Check sheet for the modelled part. Datum: model origin and axes. Units: mm. A direction names the side the tool comes from. Round coordinates to 2 decimals unless told otherwise and drop trailing zeros. Write each loop counter-clockwise with the first axis right and the second up, starting at its lowest first coordinate (ties: lowest second). Pieces come first, ordered by that corner, then holes. Notation, with made-up numbers: M 5.25,54.5 L 30.25,54.5 A17 cw 30.25,82.5 Z; hole C 83.25,40.5 d9. An arc over 180 degrees is marked long. One line per item, written item: value.
from build123d import *

# Parameters (mm, degrees)
F0_W          = 28.3
F0_H          = 28.2685337434
F0_R          = 1.5
F1_DEPTH      = 5
F2_W          = 45
F2_H          = 10
F3_DEPTH      = 5
F4_W          = 10
F4_H          = 25
F5_DEPTH      = 35
F7_DEPTH      = 30
F7_DEPTH_BACK = 10
F8_T1_DEPTH   = 51.2903171605
F8_T3_DEPTH   = 50.8819045103
F8_T5_DEPTH   = 44.5915873497
F8_T7_DEPTH   = 15.5291427062
F8_T9_DEPTH   = 33.4838731358
F8_T11_DEPTH  = 29.4646352493
F8_T13_DEPTH  = 15
F8_T15_DEPTH  = 17.5
F8_T20_DEPTH  = 5
F8_T26_DEPTH  = 5
F8_S31_W      = 5
F8_S31_H      = 5
F8_T32_DEPTH  = 5
F8_S37_W      = 5
F8_S37_H      = 5
F8_T38_DEPTH  = 5


# Not quite as in the source:
# - a fillet or chamfer that OpenCascade refuses, or shapes differently, is made with other operations: its cross-section is extruded or revolved along the edge and cut away or added


with BuildPart() as f1:
    # F0 (on Top) → F1 (new body)
    with BuildSketch(Plane.XY):
        Rectangle(F0_W, F0_H)
        with Locations((-10.4845586502, -10.7272564019)):
            Circle(F0_R, mode=Mode.SUBTRACT)
        with Locations((10.7272564019, -10.4845586502)):
            Circle(F0_R, mode=Mode.SUBTRACT)
        with Locations((-10.7272564019, 10.4845586502)):
            Circle(F0_R, mode=Mode.SUBTRACT)
        with Locations((10.4845586502, 10.7272564019)):
            Circle(F0_R, mode=Mode.SUBTRACT)
    extrude(amount=F1_DEPTH)

    # F2 (on face) → F3 (join)
    with BuildSketch(Plane.XY.offset(5)):
        with Locations((8.35, 0)):
            Rectangle(F2_W, F2_H)
    extrude(amount=F3_DEPTH)

    # F4 (on face) → F5 (join)
    with BuildSketch(Plane(origin=(0, 0, 5), x_dir=(1, 0, 0), z_dir=(0, 0, -1))):
        with Locations((25.85, 0)):
            Rectangle(F4_W, F4_H)
    extrude(amount=-F5_DEPTH)

    # F6 (on face) → F7 (join, two sides)
    with BuildSketch(Plane(origin=(20.85, 0, 0), x_dir=(0, -1, 0), z_dir=(-1, 0, 0))) as f7_sk:
        Polygon((-12.5, 50), (-12.5, 40), (12.5, 40), (12.5, 43.3012701892), align=None)
    extrude(amount=F7_DEPTH)
    extrude(f7_sk.sketch, amount=-F7_DEPTH_BACK)

    # F8: fillet of radius 5 on 9 edges, made by hand

    # F8_s2 → F8_t1 (cut)
    with BuildSketch(Plane.YZ.offset(-25.4403171605)):
        with BuildLine():
            ThreePointArc((6.2059047745, 48.3135022672), (10.543807145, 47.4506398373), (12.5, 43.4838731358))
            Line((12.5, 43.4838731358), (12.5, 50))
            Line((12.5, 50), (6.2059047745, 48.3135022672))
        make_face()
    extrude(amount=F8_T1_DEPTH, mode=Mode.SUBTRACT)

    # F8_s4 → F8_t3 (cut)
    with BuildSketch(Plane(origin=(0, -12.911414055, -3.4596029692), x_dir=(1, 0, 0), z_dir=(0, 0.9659258263, 0.2588190451))):
        with BuildLine():
            ThreePointArc((-9.15, -40.0610532507), (-7.6855339059, -43.5965871566), (-4.15, -45.0610532507))
            Line((-4.15, -45.0610532507), (-9.15, -45.0610532507))
            Line((-9.15, -45.0610532507), (-9.15, -40.0610532507))
        make_face()
    extrude(amount=F8_T3_DEPTH, mode=Mode.SUBTRACT)

    # F8_s6 → F8_t5 (cut)
    with BuildSketch(Plane.YZ.offset(-18.7415873497)):
        with BuildLine():
            ThreePointArc((-12.5, 39.4646352493), (-11.4667667015, 42.5084423944), (-8.7940952255, 44.2942643808))
            Line((-8.7940952255, 44.2942643808), (-12.5, 43.3012701892))
            Line((-12.5, 43.3012701892), (-12.5, 39.4646352493))
        make_face()
    extrude(amount=F8_T5_DEPTH, mode=Mode.SUBTRACT)

    # F8_s8 → F8_t7 (cut)
    with BuildSketch(Plane(origin=(0, 2.8685635481, 0.7686292862), x_dir=(1, 0, 0), z_dir=(0, 0.9659258263, 0.2588190451))):
        with BuildLine():
            ThreePointArc((25.85, -45.0610532507), (29.3855339059, -43.5965871566), (30.85, -40.0610532507))
            Line((30.85, -40.0610532507), (30.85, -45.0610532507))
            Line((30.85, -45.0610532507), (25.85, -45.0610532507))
        make_face()
    extrude(amount=F8_T7_DEPTH, mode=Mode.SUBTRACT)

    # F8_s10 → F8_t9 (cut)
    with BuildSketch(Plane.XY.offset(10)):
        with BuildLine():
            ThreePointArc((30.85, 7.5), (29.3855339059, 11.0355339059), (25.85, 12.5))
            Line((25.85, 12.5), (30.85, 12.5))
            Line((30.85, 12.5), (30.85, 7.5))
        make_face()
    extrude(amount=F8_T9_DEPTH, mode=Mode.SUBTRACT)

    # F8_s12 → F8_t11 (cut)
    with BuildSketch(Plane.XY.offset(10)):
        with BuildLine():
            ThreePointArc((25.85, -12.5), (29.3855339059, -11.0355339059), (30.85, -7.5))
            Line((30.85, -7.5), (30.85, -12.5))
            Line((30.85, -12.5), (25.85, -12.5))
        make_face()
    extrude(amount=F8_T11_DEPTH, mode=Mode.SUBTRACT)

    # F8_s14 → F8_t13 (cut)
    with BuildSketch(Plane.XZ.offset(-7.5)):
        with BuildLine():
            ThreePointArc((30.85, 10), (29.3855339059, 6.4644660941), (25.85, 5))
            Line((25.85, 5), (30.85, 5))
            Line((30.85, 5), (30.85, 10))
        make_face()
    extrude(amount=F8_T13_DEPTH, mode=Mode.SUBTRACT)

    # F8_s16 → F8_t15 (cut)
    with BuildSketch(Plane.YZ.offset(8.35)):
        with BuildLine():
            ThreePointArc((12.5, 10), (11.0355339059, 6.4644660941), (7.5, 5))
            Line((7.5, 5), (12.5, 5))
            Line((12.5, 5), (12.5, 10))
        make_face()
        with BuildLine():
            ThreePointArc((-12.5, 10), (-11.0355339059, 6.4644660941), (-7.5, 5))
            Line((-7.5, 5), (-12.5, 5))
            Line((-12.5, 5), (-12.5, 10))
        make_face()
    extrude(amount=F8_T15_DEPTH, mode=Mode.SUBTRACT)


with BuildPart() as f8_tool18:
    # F8_s19 → F8_t20 (new body)
    with BuildSketch(Plane.YZ.offset(25.85)):
        Polygon((7.5, 43.4838731358), (12.5, 43.4838731358), (12.5, 50), (6.2059047745, 48.3135022672), align=None)
    extrude(amount=F8_T20_DEPTH)

    # F8_s21 → F8_t22 (revolve, cut)
    with BuildSketch(Plane(origin=(25.85, 7.5, 43.4838731358), x_dir=(0, -0.608761429, -0.7933533403), z_dir=(0, -0.7933533403, 0.608761429))):
        with BuildLine():
            ThreePointArc((0, -5), (5, 0), (0, 5))
            Line((0, 5), (0, -5))
        make_face()
    revolve(axis=Axis((25.85, 7.5, 43.4838731358), (1, 0, 0)), mode=Mode.SUBTRACT)


with BuildPart() as f1_1:
    add(f1.part)

    # F8_t17: cut F8_tool18
    add(f8_tool18.part, mode=Mode.SUBTRACT)


with BuildPart() as f8_tool24:
    # F8_s25 → F8_t26 (new body)
    with BuildSketch(Plane.YZ.offset(25.85)):
        Polygon((-7.5, 39.4646352493), (-12.5, 39.4646352493), (-12.5, 43.3012701892), (-8.7940952255, 44.2942643808), align=None)
    extrude(amount=F8_T26_DEPTH)

    # F8_s27 → F8_t28 (revolve, cut)
    with BuildSketch(Plane(origin=(25.85, -7.5, 39.4646352493), x_dir=(0, 0.7933533403, -0.608761429), z_dir=(0, -0.608761429, -0.7933533403))):
        with BuildLine():
            ThreePointArc((0, -5), (5, 0), (0, 5))
            Line((0, 5), (0, -5))
        make_face()
    revolve(axis=Axis((25.85, -7.5, 39.4646352493), (1, 0, 0)), mode=Mode.SUBTRACT)


with BuildPart() as f1_2:
    add(f1_1.part)

    # F8_t23: cut F8_tool24
    add(f8_tool24.part, mode=Mode.SUBTRACT)


with BuildPart() as f8_tool30:
    # F8_s31 → F8_t32 (new body)
    with BuildSketch(Plane.XZ.offset(-7.5)):
        with Locations((28.35, 7.5)):
            Rectangle(F8_S31_W, F8_S31_H)
    extrude(amount=-F8_T32_DEPTH)

    # F8_s33 → F8_t34 (revolve, cut)
    with BuildSketch(Plane(origin=(25.85, 7.5, 10), x_dir=(-0.7071067812, 0, 0.7071067812), z_dir=(-0.7071067812, 0, -0.7071067812))):
        with BuildLine():
            ThreePointArc((0, -5), (5, 0), (0, 5))
            Line((0, 5), (0, -5))
        make_face()
    revolve(axis=Axis((25.85, 7.5, 10), (0, 1, 0)), mode=Mode.SUBTRACT)


with BuildPart() as f1_3:
    add(f1_2.part)

    # F8_t29: cut F8_tool30
    add(f8_tool30.part, mode=Mode.SUBTRACT)


with BuildPart() as f8_tool36:
    # F8_s37 → F8_t38 (new body)
    with BuildSketch(Plane.XY.offset(10)):
        with Locations((28.35, -10)):
            Rectangle(F8_S37_W, F8_S37_H)
    extrude(amount=-F8_T38_DEPTH)

    # F8_s39 → F8_t40 (revolve, cut)
    with BuildSketch(Plane(origin=(25.85, -7.5, 10), x_dir=(-0.7071067812, 0.7071067812, 0), z_dir=(-0.7071067812, -0.7071067812, 0))):
        with BuildLine():
            ThreePointArc((0, -5), (5, 0), (0, 5))
            Line((0, 5), (0, -5))
        make_face()
    revolve(axis=Axis((25.85, -7.5, 10), (0, 0, -1)), mode=Mode.SUBTRACT)


with BuildPart() as f1_4:
    add(f1_3.part)

    # F8_t35: cut F8_tool36
    add(f8_tool36.part, mode=Mode.SUBTRACT)


solid = f1_4.part
Q1. Sectioned sample at D-D on x = -5.5. Enter the section's corners in (y, z).
Completed:
outline: M -14.13,0 L 14.13,0 L 14.13,5 L 5,5 L 5,10 L -5,10 L -5,5 L -14.13,5 Z; M -12.47,40 L 12.5,40 L 12.5,43.48 A5 ccw 7.56,48.48 L -10.05,43.77 A5 ccw Z
Q2. Access from +Z, -Z, +X, -X, +Y, -Y to the whole of each face (thin tool, end or side, straight path). Record for faces 1 (the flat face through (14.15, 0, 2)), 2 (the flat face through (0, -10, 5)), 3 (the cylindrical face through (11.291, 11.992, 2.465)).
Completed:
face 1: -Z, +X, +Y, -Y
face 2: -X, -Y
face 3: -Z
Q3. Sectioned sample at A-A on x = 4. Enter the section's corners in (y, z), and give its area (3 significant figures).
Completed:
outline: M -14.13,0 L 14.13,0 L 14.13,5 L 5,5 L 5,10 L -5,10 L -5,5 L -14.13,5 Z; M -12.47,40 L 12.5,40 L 12.5,43.48 A5 ccw 6.21,48.31 L -8.79,44.29 A5 ccw Z
area: 345 mm^2
Q4. Sectioned sample at B-B on x = 11. Enter the section's corners in (y, z).
Completed:
outline: M -14.13,0 L -11.96,0 L -11.96,5 L -14.13,5 Z; M -12.47,40 L 12.5,40 L 12.5,43.48 A5 ccw 6.21,48.31 L -8.79,44.29 A5 ccw Z; M -9.01,0 L 9.32,0 L 9.32,5 L 5,5 L 5,10 L -5,10 L -5,5 L -9.01,5 Z; M 12.14,0 L 14.13,0 L 14.13,5 L 12.14,5 Z
Q5. Scan lines: line 1 (X direction, y = 8.5, z = 3); line 2 (Z direction, x = -2, y = -12.75); line 3 (Y direction, x = 24, z = 36). Record each from-to range of solid material in increasing order. Write a range as [from, to].
Completed:
line 1: [-14.15, 14.15]
line 2: [0, 5]
line 3: [-12.5, 12.5]
Q6. Draft check along X on faces 4 (the flat face through (-9.15, 6, 42)), 5 (the flat face through (6, 0, 40)), 6 (the cylindrical face through (-11.983, -10.661, 2.465)). Enter one of: pulls with the +X half, pulls with the -X half, needs draft (parallel to the pull), parting line crosses it, or undercut.
Completed:
face 4: pulls with the -X half
face 5: needs draft
face 6: undercut
Q7. Depth check by flat-ended pin: P1, Ø10, axis at y = -1, z = 29, coming from the -X side; P2, Ø6, axis at x = 21, y = 0, coming from the -Z side; P3, Ø3.5, axis at x = -10.48, y = -10.73, coming from the +Z side. Enter the tip coordinate at first touch or a pass-through.
Completed:
P1: x = 20.85
P2: z = 5
P3: z = 40.7
Q8. Sectioned sample at C-C on z = 6. Enter the section's corners in (x, y), and give its area (3 significant figures).
Completed:
outline: M -14.15,-5 L 20.85,-5 L 20.85,-10.5 L 25.85,-10.5 A3 ccw 28.85,-7.5 L 28.85,7.5 A3 ccw 25.85,10.5 L 20.85,10.5 L 20.85,5 L -14.15,5 Z
area: 514 mm^2
